from build123d import *

# Parameters (mm, degrees)
SKETCH_1_W      = 600
SKETCH_1_H      = 430
EXTRUDE_1_DEPTH = 195
SKETCH_2_W      = 520
SKETCH_2_H      = 350
EXTRUDE_2_DEPTH = 120
SKETCH_3_W      = 635
SKETCH_3_H      = 430
EXTRUDE_3_DEPTH = 325
FILLET_2_R      = 10
FILLET_3_R      = 10


with BuildPart() as part:
    # 草圖1 → 填料-伸長1 (new body)
    with BuildSketch(Plane(origin=(0, 0, 0), x_dir=(1, 0, 0), z_dir=(0, 1, 0))):
        Rectangle(SKETCH_1_W, SKETCH_1_H)
    extrude(amount=EXTRUDE_1_DEPTH)

    # 草圖2 → 填料-伸長2 (add)
    with BuildSketch(Plane(origin=(0, 195, 0), x_dir=(1, 0, 0), z_dir=(0, 1, 0))):
        Rectangle(SKETCH_2_W, SKETCH_2_H)
    extrude(amount=EXTRUDE_2_DEPTH)

    # 草圖3 → 填料-伸長3 (add)
    with BuildSketch(Plane(origin=(0, 315, 0), x_dir=(1, 0, 0), z_dir=(0, 1, 0))):
        Rectangle(SKETCH_3_W, SKETCH_3_H)
    extrude(amount=EXTRUDE_3_DEPTH)

    # 圓角2
    fillet_2_edges = [part.edges().sort_by_distance(p)[0] for p in [
        (317.5, 477.5, 215),
        (317.5, 477.5, -215),
        (-317.5, 477.5, -215),
        (-317.5, 477.5, 215),
    ]]
    fillet(fillet_2_edges, radius=FILLET_2_R)

    # 圓角3
    fillet_3_edges = [part.edges().sort_by_distance(p)[0] for p in [
        (300, 97.5, 215),
        (-300, 97.5, 215),
        (-300, 97.5, -215),
        (300, 97.5, -215),
    ]]
    fillet(fillet_3_edges, radius=FILLET_3_R)


solid = part.part
Model file for the job. Use its own axes, mm. A direction names the side the tool comes from. Round coordinates to 2 decimals unless told otherwise and drop trailing zeros. Order: outer loops, then holes, each group sorted by start corner. A loop starts at its lowest first (then second) coordinate and runs counter-clockwise, first axis right, second up.
(1) Pin check, flat tips, straight feed: pin 1 (1 mm diameter, centred on y = 144, z = 112.5, fed in from -X); pin 2 (12 mm diameter, centred on x = -137.5, y = 235, fed in from -Z); pin 3 (1 mm diameter, centred on x = 98, y = 248, fed in from +Z). Stop position of each tip, or through.
(2) Band-saw the part on B-B (x = 184.5). List the corners of the cut face in (y, z).
(3) Drill centre lines: line 1 (Y direction, x = 266.5, z = 47); line 2 (Z direction, x = 58, y = 195.5); line 3 (X direction, y = 60.5, z = 22). Where is each one in solid material? Low to high.
(4) 3-axis set-ups, long thin cutter, end or side, ignore diameter. For faces 1 (the face through (-4, 195, 188)), 2 (the face through (-4, 254, 175)), 3 (the face through (300, 96, 3)), 4 (the face through (-4, 254, -175)), 5 (the face through (-260, 254, 2)): which of +Z, -Z, +X, -X, +Y, -Y reach the whole face in a straight line?
(5) Band-saw the part on C-C (y = 204.5). List the corners of the cut face in (x, z), then the cut area to 3 significant figures.
(6) Band-saw the part on A-A (z = 68). List the corners of the cut face in (x, y), then the cut area to 3 significant figures.
(7) Pull direction Y, two halves, no side cores. Call faces 6 (the face through (260, 254, 2)), 7 (the face through (-4, 315, 188)), 8 (the face through (-4, 640, -3)), 9 (the face through (-317.5, 475, 3)): released by +Y, released by -Y, zero draft, split by the parting line, or undercut.
Verdict:
1. pin 1: stops at x = -300
1. pin 2: stops at z = -175
1. pin 3: stops at z = 175
2. outline: (0, -215) - (195, -215) - (195, -175) - (315, -175) - (315, -215) - (640, -215) - (640, 215) - (315, 215) - (315, 175) - (195, 175) - (195, 215) - (0, 215) - close
3. line 1: y = 0 to 195, 315 to 640
3. line 2: z = -175 to 175
3. line 3: x = -300 to 300
4. face 1: none
4. face 2: +Z, +X, -X
4. face 3: +Z, -Z, +X, -Y
4. face 4: -Z, +X, -X
4. face 5: +Z, -Z, -X
5. outline: (-260, -175) - (260, -175) - (260, 175) - (-260, 175) - close
5. area: 182,000 mm2
6. outline: (-317.5, 315) - (-260, 315) - (-260, 195) - (-300, 195) - (-300, 0) - (300, 0) - (300, 195) - (260, 195) - (260, 315) - (317.5, 315) - (317.5, 640) - (-317.5, 640) - close
6. area: 386,000 mm2
7. face 6: undercut
7. face 7: undercut
7. face 8: released by +Y
7. face 9: zero draft
